Source: CAD feature listing. Evaluate the final solid. Frame: model axes, mm. Give positions to 0.01 mm unless a question says otherwise; leave off trailing zeros. Write each loop counter-clockwise with the first axis right and the second up, starting at its lowest first coordinate (ties: lowest second). Pieces come first, ordered by that corner, then holes.
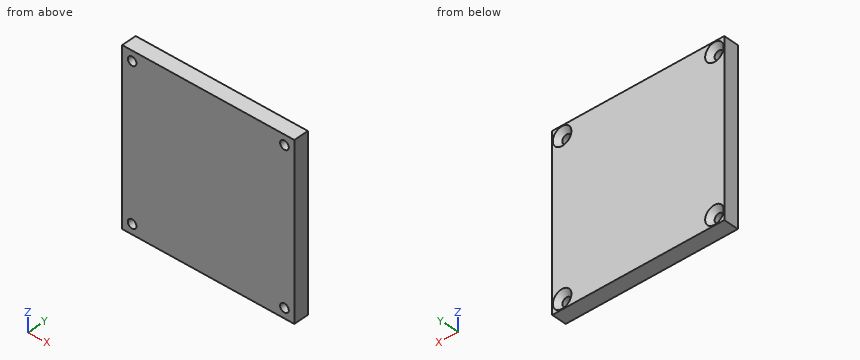
Autodesk Inventor part; units mm, degrees
ref_plane "YZ Plane" through (0, 0, 0) normal (1, 0, 0) x (0, 1, 0)
ref_plane "XZ Plane" through (0, 0, 0) normal (0, 1, 0) x (-1, 0, 0)
ref_plane "XY Plane" through (0, 0, 0) normal (0, 0, 1) x (1, 0, 0)
sketch "Sketch1" plane through (0, 0, 0) normal (0, 1, 0) x (-1, 0, 0)
  line L0 (34.75, -34.75) -> (-34.75, -34.75)
  line L1 (-34.75, -34.75) -> (-34.75, 34.75)
  line L2 (-34.75, 34.75) -> (34.75, 34.75)
  line L3 (34.75, 34.75) -> (34.75, -34.75)
  line L4 (34.75, -34.75) -> (-34.75, 34.75) construction
  line L5 (-34.75, -34.75) -> (34.75, 34.75) construction
  circle A0 centre (30.75, 30.75) radius 1.75
  circle A1 centre (30.75, -30.75) radius 1.75
  circle A2 centre (-30.75, 30.75) radius 1.75
  circle A3 centre (-30.75, -30.75) radius 1.75
  point P0 (0, 0)
  dimension "d0" = 69.5
  dimension "d1" = 69.5
  dimension "d2" = 3.5
  dimension "d3" = 4
  dimension "d4" = 3.5
  dimension "d5" = 4
  dimension "d6" = 3.5
  dimension "d7" = 3.5
  dimension "d8" = 4
  dimension "d14" = 4
extrude "Extrusion1" add sketch "Sketch1" along normal blind 6
chamfer "Chamfer1" distance 2 angle 45 4 edges at (-29, 6, 30.75) (-29, 6, -30.75) (32.5, 6, 30.75) (32.5, 6, -30.75)
equation "\"d1\" = d0"
equation "\"d4\" = d2"
equation "\"d5\" = d3"
equation "\"d6\" = d2"
equation "\"d7\" = d2"
equation "\"d8\" = d3"
equation "\"d14\" = d3"
properties part number "Modulo"
1. Cut plane A-A, the plane z = 30.75. Return the cut outline in (x, y).
2. Cut plane C-C, the plane x = -30.75. Return the cut outline in (y, z), then the cut area to 3 significant figures.
3. Line query: L1, parallel to Z at x = -30.75, y = 0.9. Output: solid intervals per line, ascending.
4. Contact query for a flat-ended pin moving along its axis: P1, Ø4, axis at x = 30.75, z = -30.75, coming from the +Y side. Output: stop coordinate, or through.
5. Cut plane B-B, the plane y = 4.8. Return the cut outline in (x, z), then the cut area to 3 significant figures.
Response values:
1. outline: (-34.75, 0) - (-32.5, 0) - (-32.5, 4) - (-34.5, 6) - (-34.75, 6) - close; (-29, 0) - (29, 0) - (29, 4) - (27, 6) - (-27, 6) - (-29, 4) - close; (32.5, 0) - (34.75, 0) - (34.75, 6) - (34.5, 6) - (32.5, 4) - close
2. outline: (0, -34.75) - (6, -34.75) - (6, -34.5) - (4, -32.5) - (0, -32.5) - close; (0, -29) - (4, -29) - (6, -27) - (6, 27) - (4, 29) - (0, 29) - close; (0, 32.5) - (4, 32.5) - (6, 34.5) - (6, 34.75) - (0, 34.75) - close
2. area: 367 mm2
3. L1: z = -34.75 to -32.5, -29 to 29, 32.5 to 34.75
4. P1: stops at y = 4.25
5. outline: (-34.75, -34.75) - (34.75, -34.75) - (34.75, 34.75) - (-34.75, 34.75) - close; hole circle Ø5.1 at (-30.75, -30.75); hole circle Ø5.1 at (-30.75, 30.75); hole circle Ø5.1 at (30.75, -30.75); hole circle Ø5.1 at (30.75, 30.75)
5. area: 4,750 mm2
